Part print with two shaded views. Sizes in mm from the minimum x, y, z corner. A direction names the side the tool comes from. Round coordinates to 2 decimals unless told otherwise and drop trailing zeros. Order: outer loops, then holes, each group sorted by start corner. A loop starts at its lowest first (then second) coordinate and runs counter-clockwise, first axis right, second up. Notation, with made-up numbers: (55.25, 88) -> (61.25, 88) arc R16 cw to (61.25, 107) -> close; hole circle Ø2 at (-35, 61). An arc over 180 degrees is marked (long way). Use a Markdown table: item, result. Add a question column.
Item 1: Two-plate mould, pull along X, no slides. Class the marked faces 1, 2 and 3: released by +X, released by -X, zero draft, split by the parting line, or undercut.
Item 2: Probe L1, parallel to Y at x = 35, z = 23.5; L2, parallel to Z at x = 64.5, y = 50; L3, parallel to X at y = 61, z = 70. List the from-to ranges inside material, lowest first.
Item 3: Slice it at C-C, the plane x = 35. Give the cut face in (y, z), plus the area to 3 significant figures.
Item 4: Slice it at A-A, the plane y = 73.5. Give the cut face in (x, z), plus the area to 3 significant figures.
Item 5: Pin check, flat tips, straight feed: pin 1 (5 mm diameter, centred on x = 51, y = 27, fed in from +Z); pin 2 (9 mm diameter, centred on y = 50, z = 96, fed in from -X); pin 3 (3.5 mm diameter, centred on x = 65, y = 26.5, fed in from +Z); pin 4 (5 mm diameter, centred on x = 65.5, z = 86.5, fed in from +Y). Stop position of each tip, or through.
Item 6: Slice it at D-D, the plane y = 50. Give the cut face in (x, z).
Item 7: 3-axis set-ups, long thin cutter, end or side, ignore diameter. For the marked faces 4, 5, 6 and 7: which of +Z, -Z, +X, -X, +Y, -Y reach the whole face in a straight line?
Item 8: Slice it at B-B, the plane z = 40. Give the cut face in (x, y), plus the area to 3 significant figures.
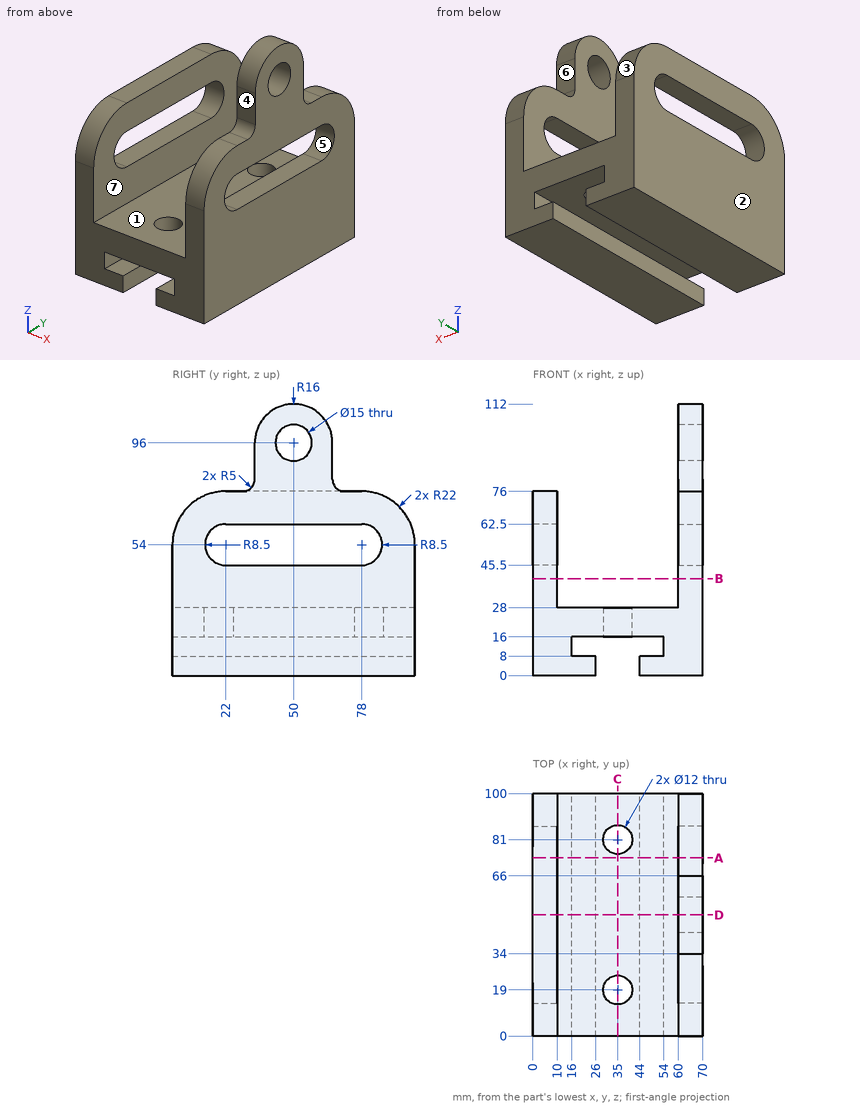
Check sheet entries:
| question | item | result |
|---|---|---|
| 1 | face 1 | undercut |
| 1 | face 2 | released by -X |
| 1 | face 3 | zero draft |
| 2 | L1 | 0 to 13, 25 to 75, 87 to 100 |
| 2 | L2 | 0 to 45.5, 62.5 to 88.5, 103.5 to 112 |
| 2 | L3 | 0 to 10, 60 to 70 |
| 3 | outline | (0, 16) -> (13, 16) -> (13, 28) -> (0, 28) -> close; (25, 16) -> (75, 16) -> (75, 28) -> (25, 28) -> close; (87, 16) -> (100, 16) -> (100, 28) -> (87, 28) -> close |
| 3 | area | 912 mm2 |
| 4 | outline | (0, 0) -> (26, 0) -> (26, 8) -> (16, 8) -> (16, 16) -> (54, 16) -> (54, 8) -> (44, 8) -> (44, 0) -> (70, 0) -> (70, 45.5) -> (60, 45.5) -> (60, 28) -> (10, 28) -> (10, 45.5) -> (0, 45.5) -> close; (0, 62.5) -> (10, 62.5) -> (10, 76) -> (0, 76) -> close; (60, 62.5) -> (70, 62.5) -> (70, 76) -> (60, 76) -> close |
| 4 | area | 2,130 mm2 |
| 5 | pin 1 | z = 28 |
| 5 | pin 2 | through |
| 5 | pin 3 | z = 76 |
| 5 | pin 4 | y = 66 |
| 6 | outline | (0, 0) -> (26, 0) -> (26, 8) -> (16, 8) -> (16, 16) -> (54, 16) -> (54, 8) -> (44, 8) -> (44, 0) -> (70, 0) -> (70, 45.5) -> (60, 45.5) -> (60, 28) -> (10, 28) -> (10, 45.5) -> (0, 45.5) -> close; (0, 62.5) -> (10, 62.5) -> (10, 76) -> (0, 76) -> close; (60, 62.5) -> (70, 62.5) -> (70, 88.5) -> (60, 88.5) -> close; (60, 103.5) -> (70, 103.5) -> (70, 112) -> (60, 112) -> close |
| 7 | face 4 | +Z, +X, -X, -Y |
| 7 | face 5 | +X, -X |
| 7 | face 6 | +Z, +X, -X, +Y |
| 7 | face 7 | +Z, +Y, -Y |
| 8 | outline | (0, 0) -> (10, 0) -> (10, 100) -> (0, 100) -> close; (60, 0) -> (70, 0) -> (70, 100) -> (60, 100) -> close |
| 8 | area | 2,000 mm2 |
